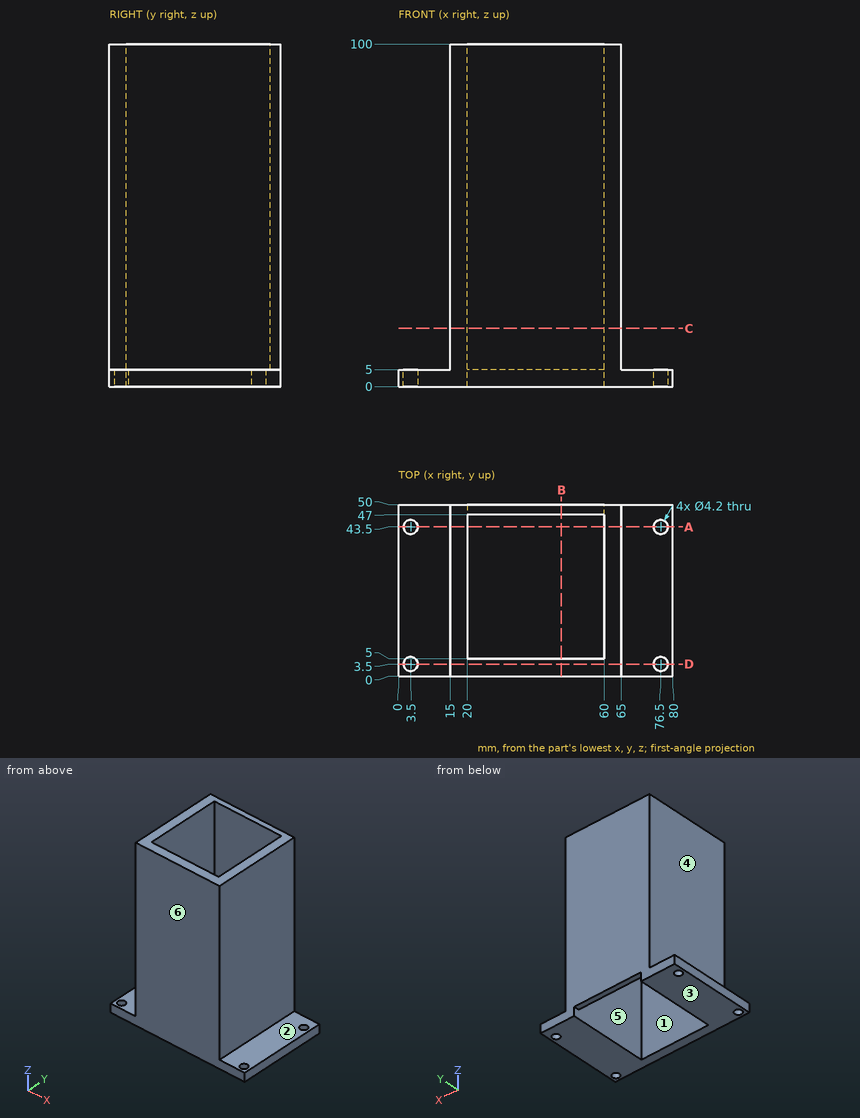
The figure shows three views and two pictorial views of one solid part (mm, origin at its lowest corner). Answer the questions. A direction names the side the tool comes from. Give positions to 0.01 mm unless a question says otherwise; leave off trailing zeros. Write each loop counter-clockwise with the first axis right and the second up, starting at its lowest first coordinate (ties: lowest second). Pieces come first, ordered by that corner, then holes.
Q1. The part is cut by section D-D on y = 3.5. Give the vertices of the cut face in (x, z), and give its area (3 significant figures).
Answer:
outline: (0, 0) - (1.4, 0) - (1.4, 5) - (0, 5) - close; (5.6, 0) - (74.4, 0) - (74.4, 5) - (65, 5) - (65, 100) - (15, 100) - (15, 5) - (5.6, 5) - close; (78.6, 0) - (80, 0) - (80, 5) - (78.6, 5) - close
area: 5,110 mm2
Q2. A tool of negligible diameter and unlimited length cuts with its end or side. For the marked faces 1, 2 and 3, from which of +Z, -Z, +X, -X, +Y, -Y can it reach the whole face along a straight path? Write none if from no direction.
Answer:
face 1: +Z, -Z
face 2: +Z, +X, +Y, -Y
face 3: -Z, +X, -X, +Y, -Y
Q3. The part is cut by section C-C on z = 17. Give the vertices of the cut face in (x, y), and give its area (3 significant figures).
Answer:
outline: (15, 0) - (65, 0) - (65, 50) - (15, 50) - close; hole (20, 5) - (60, 5) - (60, 47) - (20, 47) - close
area: 820 mm2
Q4. The part is cut by section B-B on x = 47.5. Give the vertices of the cut face in (y, z), and give its area (3 significant figures).
Answer:
outline: (0, 0) - (5, 0) - (5, 100) - (0, 100) - close; (47, 5) - (50, 5) - (50, 100) - (47, 100) - close
area: 785 mm2
Q5. For a pull along Y with two mould halves and no side action, classify the marked faces 4, 5 and 6 as released by +Y, released by -Y, zero draft, split by the parting line, or undercut.
Answer:
face 4: zero draft
face 5: undercut
face 6: released by -Y
Q6. Straight lines are drawn through the part: L1, parallel to Y at x = 3.5, z = 2.1; L2, parallel to X at y = 43.5, z = 3; L3, parallel to X at y = 18.5, z = 91.5. For each, find the intervals that lie inside material, in ascending order.
Answer:
L1: y = 0 to 1.4, 5.6 to 41.4, 45.6 to 50
L2: x = 0 to 1.4, 5.6 to 20, 60 to 74.4, 78.6 to 80
L3: x = 15 to 20, 60 to 65
Q7. Given pin 1 (2 mm diameter, centred on y = 33, z = 22, fed in from +X); pin 2 (2.5 mm diameter, centred on x = 48, y = 49, fed in from -Z); pin 3 (15 mm diameter, centred on y = 20, z = 45, fed in from -X), each flat-ended and moving along its own axis, determine where each tip first touches the part or whether it passes through.
Answer:
pin 1: stops at x = 65
pin 2: stops at z = 5
pin 3: stops at x = 15
Q8. The part is cut by section A-A on y = 43.5. Give the vertices of the cut face in (x, z), and give its area (3 significant figures).
Answer:
outline: (0, 0) - (1.4, 0) - (1.4, 5) - (0, 5) - close; (5.6, 0) - (20, 0) - (20, 100) - (15, 100) - (15, 5) - (5.6, 5) - close; (60, 0) - (74.4, 0) - (74.4, 5) - (65, 5) - (65, 100) - (60, 100) - close; (78.6, 0) - (80, 0) - (80, 5) - (78.6, 5) - close
area: 1,110 mm2
